Drawing for the job (mm, zero at the part's lowest x, y, z). Round coordinates to 2 decimals unless told otherwise and drop trailing zeros. Write each loop counter-clockwise with the first axis right and the second up, starting at its lowest first coordinate (ties: lowest second). Pieces come first, ordered by that corner, then holes.
Item 1: Wall check: probe 1 along Y at (x, z) = (7.75, 3.3); probe 2 along Y at (x, z) = (7.75, 7.95); probe 3 along X at (y, z) = (8.75, 1.5) (1 decimal). Give the ranges that are in metal, low to high.
Item 2: Band-saw the part on D-D, the plane z = 7.5. Write the cut outline in (x, y), then the cut area to 3 significant figures.
Item 3: Mould opens along Z. For the marked faces 1, 2, 3 and 4 say: +Z half, -Z half, draft (parallel to the pull), parting line (faces both ways), or undercut.
Item 4: Drop flat-ended pins along their axis: pin 1 Ø5 at (y, z) = (4, 2) entering from +X; pin 2 Ø1 at (y, z) = (7, 6.5) entering from +X; pin 3 Ø5 at (x, z) = (13.5, 1.5) entering from -Y. Give the stop position or say it passes through.
Item 5: Band-saw the part on C-C, the plane z = 4.75. Write the cut outline in (x, y), then the cut area to 3 significant figures.
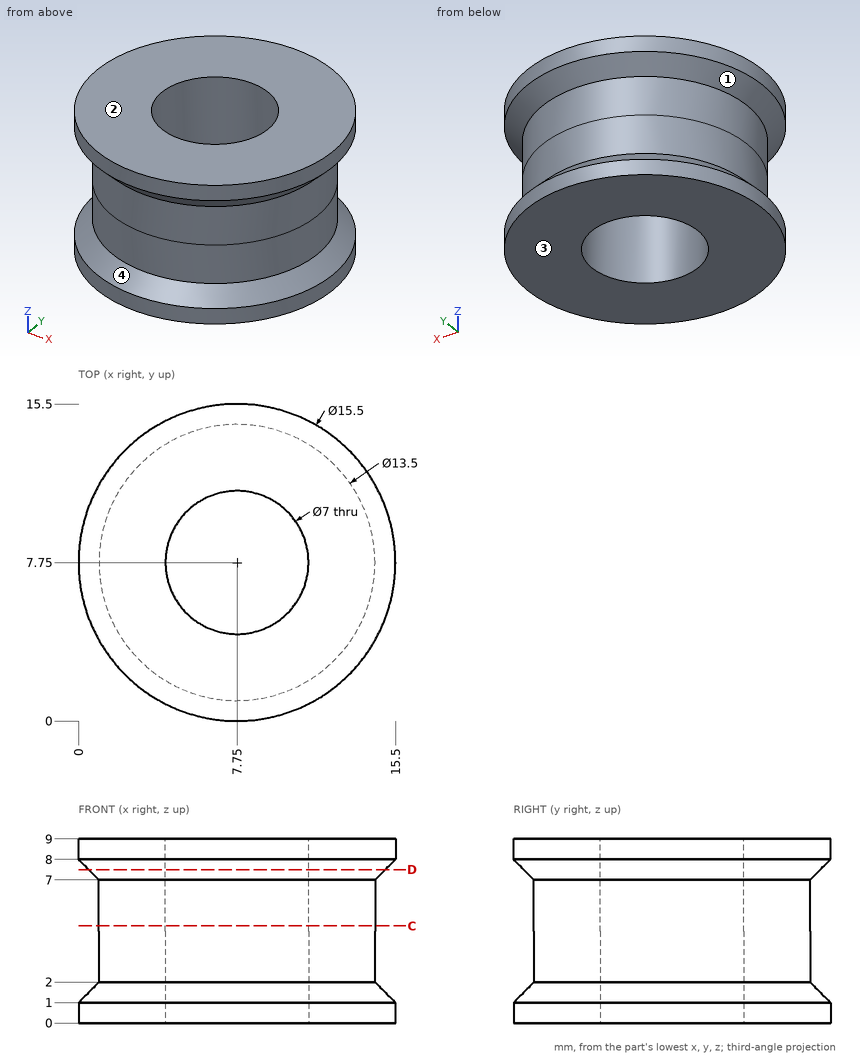
Results:
1. probe 1: y = 1 to 4.25, 11.25 to 14.5
1. probe 2: y = 0.05 to 4.25, 11.25 to 15.45
1. probe 3: x = 0.6 to 4.4, 11.1 to 14.9
2. outline: circle Ø14.5 at (7.75, 7.75); hole circle Ø7 at (7.75, 7.75)
2. area: 127 mm2
3. face 1: undercut
3. face 2: +Z half
3. face 3: -Z half
3. face 4: undercut
4. pin 1: stops at x = 15.36
4. pin 2: stops at x = 14.5
4. pin 3: stops at y = 0.74
5. outline: circle Ø13.5 at (7.75, 7.75); hole circle Ø7 at (7.75, 7.75)
5. area: 105 mm2
